Verification items for the finished model (mm, model axes). Give positions to 0.01 mm unless a question says otherwise; leave off trailing zeros. Loops run counter-clockwise (first coordinate to the right, second up) from the corner with the lowest first, then second, coordinate; pieces in that order, holes last. Notation, with made-up numbers: (78.5, -3.75) -> (100.5, -3.75) arc R18 cw to (100.5, 6.25) -> close; hole circle Ø11 at (80.5, 86). An arc over 180 degrees is marked (long way). Answer in a Markdown table with one row per item. Add a question column.
Q1. Section check A-A on y = 11. Enter the section's corners in (x, z), and give its area (3 significant figures).
Q2. Gauge pin test, flat ends, axial feed: P1, Ø2.5, axis at x = 26, z = 1.5, coming from the -Y side; P2, Ø0.6, axis at x = 1, z = 2, coming from the +Y side; P3, Ø10.5, axis at x = 8, y = 28, coming from the +Z side. Record the tip position at first contact, or that the pin passes through.
Q3. Material ranges on probe 1 along Y at (x, z) = (38, 3.2); probe 2 along Y at (x, z) = (39, 0.65); probe 3 along X at (y, z) = (16.5, 3.5), recorded low to high.
Q4. Section check C-C on z = 3.3. Give the number of separate pieces and of enclosed holes in the cut face, and give its area (3 significant figures).
Q5. Section check D-D on x = 47.5. Enter the section's corners in (y, z).
Q6. Section check B-B on x = 39. Enter the section's corners in (y, z), and give its area (3 significant figures).
Autodesk Inventor part; units mm, degrees
ref_plane "YZ Plane" through (0, 0, 0) normal (1, 0, 0) x (0, 1, 0)
ref_plane "XZ Plane" through (0, 0, 0) normal (0, 1, 0) x (-1, 0, 0)
ref_plane "XY Plane" through (0, 0, 0) normal (0, 0, 1) x (1, 0, 0)
sketch "Sketch1" plane through (0, 0, 0) normal (0, 0, 1) x (1, 0, 0)
  line L0 (0, 0) -> (55, 0)
  line L1 (55, 0) -> (55, 80)
  line L2 (55, 80) -> (0, 80)
  line L3 (0, 80) -> (0, 0)
  dimension "d0" = 55
  dimension "d1" = 80
extrude "Extrusion1" add sketch "Sketch1" along normal blind 5
sketch "Sketch6" plane through (0, 0, 5) normal (0, 0, 1) x (1, 0, 0)
  line L0 (0, 0) -> (0, 80)
  line L1 (55, 0) -> (0, 0)
  line L2 (0, 80) -> (55, 80)
  line L3 (0, 48) -> (2, 48)
  line L4 (2, 48) -> (10.5744, 80)
  dimension "d37" = 15
  dimension "d38" = 2
  dimension "d39" = 48
extrude "Extrusion4" cut sketch "Sketch6" against normal blind 5
sketch "Sketch7" plane through (0, 0, 5) normal (0, 0, 1) x (1, 0, 0)
  line L0 (10.5744, 80) -> (2, 48)
  line L1 (55, 80) -> (55, 0)
  line L2 (10.5744, 80) -> (55, 80)
  line L3 (40, 46) -> (40, 75)
  line L4 (40, 75) -> (16.4816, 75)
  line L5 (16.4816, 75) -> (8.711, 46)
  line L6 (8.711, 46) -> (40, 46)
  dimension "d42" = 29
  dimension "d43" = 5
  dimension "d44" = 15
  dimension "d45" = 7
extrude "Extrusion5" cut sketch "Sketch7" against normal blind 5
fillet "Fillet2" radius 2.5 4 edges at (16.4816, 75, 2.5) (40, 75, 2.5) (8.711, 46, 2.5) (40, 46, 2.5)
sketch "Sketch8" plane through (0, 0, 5) normal (0, 0, 1) x (1, 0, 0)
  line L0 (0, 0) -> (0, 48)
  line L1 (55, 0) -> (0, 0)
  line L2 (55, 80) -> (55, 0)
  point P0 (8, 28)
  point P1 (39, 11)
  dimension "d49" = 8
  dimension "d50" = 16
  dimension "d51" = 28
  dimension "d52" = 11
hole "Hole3" at (8, 28, 5) at (39, 11, 5) direction (0, 0, -1) diameter 6.5 depth 5 tip angle 118 countersink diameter 11.5 countersink angle 90
sketch "Sketch9" plane through (0, 0, 0) normal (0, 0, -1) x (-1, 0, 0)
  line L0 (-55, 0) -> (-55, 80)
  line L1 (0, 0) -> (-55, 0)
  line L2 (0, 48) -> (0, 0)
  point P0 (-15.5, 16.5)
  point P1 (-47.5, 25)
  dimension "d60" = 16.5
  dimension "d61" = 15.5
  dimension "d62" = 25
  dimension "d63" = 7.5
hole "Hole4" at (15.5, 16.5, 0) at (47.5, 25, 0) direction (0, 0, 1) diameter 3.175 depth 5 tip angle 118 countersink diameter 4 countersink angle 90
properties part number "LATERAL-ESQUERDA" material "Carbon Steel"
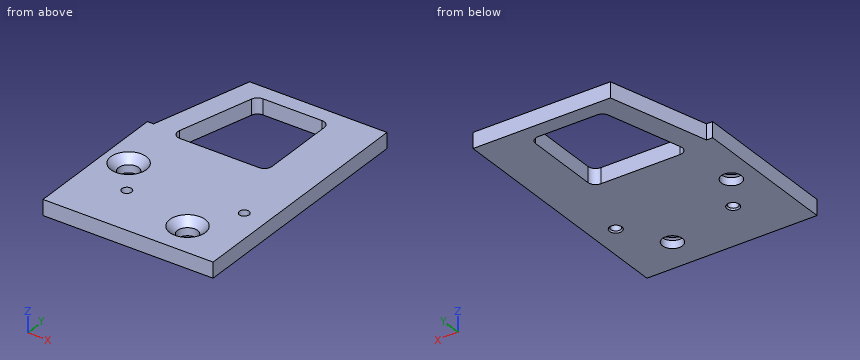
Taken from the geometry:
| question | item | result |
|---|---|---|
| 1 | outline | (0, 0) -> (35.75, 0) -> (35.75, 2.5) -> (33.25, 5) -> (0, 5) -> close; (42.25, 0) -> (55, 0) -> (55, 5) -> (44.75, 5) -> (42.25, 2.5) -> close |
| 1 | area | 236 mm² |
| 2 | P1 | stops at y = 0 |
| 2 | P2 | stops at y = 48 |
| 2 | P3 | stops at z = 4.5 |
| 3 | probe 1 | y = 0 to 7.18, 14.82 to 46.05, 74.95 to 80 |
| 3 | probe 2 | y = 0 to 7.75, 14.25 to 46.5, 74.5 to 80 |
| 3 | probe 3 | x = 0 to 13.91, 17.09 to 55 |
| 4 | separate pieces | 1 |
| 4 | enclosed holes | 5 |
| 4 | area | 3,290 mm² |
| 5 | outline | (0, 0) -> (23, 0) -> (23.41, 0.41) -> (23.41, 5) -> (0, 5) -> close; (26.59, 0.41) -> (27, 0) -> (80, 0) -> (80, 5) -> (26.59, 5) -> close |
| 6 | outline | (0, 0) -> (7.75, 0) -> (7.75, 2.5) -> (5.25, 5) -> (0, 5) -> close; (14.25, 0) -> (46.5, 0) -> (46.5, 5) -> (16.75, 5) -> (14.25, 2.5) -> close; (74.5, 0) -> (80, 0) -> (80, 5) -> (74.5, 5) -> close |
| 6 | area | 221 mm² |
